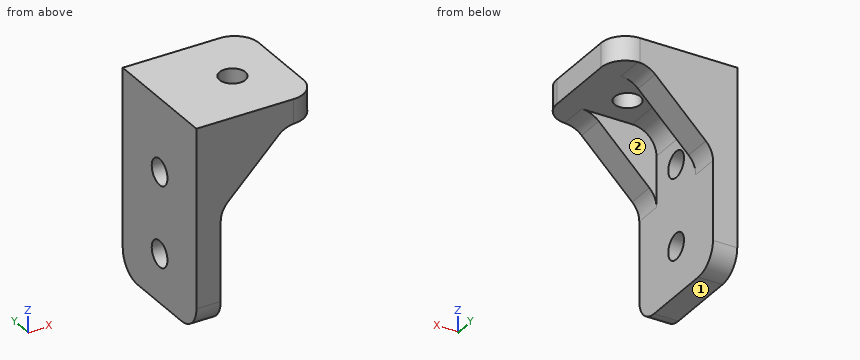
from build123d import *

# Parameters (mm, degrees)
SKETCH1_W           = 3
SKETCH1_H           = 22
SKETCH1_H_2         = 3
SKETCH1_W_2         = 12
BOSS_EXTRUDE1_DEPTH = 15
SKETCH2_R           = 1.6
CUT_EXTRUDE1_DEPTH  = 31.56141358
SKETCH3_R           = 1.6
CUT_EXTRUDE2_DEPTH  = 32.527765541
FILLET1_R           = 3
CHAMFER1_SIZE       = 8
SKETCH6_W           = 8
SKETCH6_H           = 8
CUT_EXTRUDE5_DEPTH  = 12
FILLET2_R           = 3
SKETCH7_W           = 15
SKETCH7_H           = 25
CUT_EXTRUDE6_DEPTH  = 33.787192713


with BuildPart() as part:
    # Sketch1 → Boss-Extrude1 (new body)
    with BuildSketch(Plane(origin=(0, 0, 0), x_dir=(1, 0, 0), z_dir=(0, 1, 0))):
        with Locations((1.5, 14)):
            Rectangle(SKETCH1_W, SKETCH1_H)
        with Locations((1.5, 1.5)):
            Rectangle(SKETCH1_W, SKETCH1_H_2)
        with Locations((9, 1.5)):
            Rectangle(SKETCH1_W_2, SKETCH1_H_2)
    extrude(amount=BOSS_EXTRUDE1_DEPTH)

    # Sketch2 → Cut-Extrude1 (cut, through all)
    with BuildSketch(Plane(origin=(0, 0, -3), x_dir=(-1, 0, 0), z_dir=(0, 0, -1))):
        with Locations((-9, 7.5)):
            Circle(SKETCH2_R)
    extrude(amount=-CUT_EXTRUDE1_DEPTH, mode=Mode.SUBTRACT)

    # Sketch3 → Cut-Extrude2 (cut, through all)
    with BuildSketch(Plane(origin=(3, 0, 0), x_dir=(0, 0, -1), z_dir=(1, 0, 0))):
        with Locations((9, 7.5)):
            Circle(SKETCH3_R)
        with Locations((19, 7.5)):
            Circle(SKETCH3_R)
    extrude(amount=-CUT_EXTRUDE2_DEPTH, mode=Mode.SUBTRACT)

    # Fillet1
    fillet1_edges = [part.edges().sort_by_distance(p)[0] for p in [
        (15, 15, -1.5),
        (1.5, 15, -25),
        (1.5, 0, -25),
        (15, 0, -1.5),
    ]]
    fillet(fillet1_edges, radius=FILLET1_R)

    # Chamfer1
    # the kernel refuses this chamfer: 8 mm, written as the material it adds along each edge
    with BuildSketch(Plane(origin=(3, 0, -3), x_dir=(-0.027495876610586382, 0, -0.9996219169112968), z_dir=(0, 1, 0))) as chamfer1_piece_1_section:
        Polygon((CHAMFER1_SIZE * 0.999621916911, -CHAMFER1_SIZE * 0.0274958766106), (-CHAMFER1_SIZE * 0.0274958766106, -CHAMFER1_SIZE * 0.999621916911), (0, 0), align=None)
    chamfer1_piece_1 = extrude(amount=15, mode=Mode.PRIVATE)
    chamfer1_piece_1 = chamfer1_piece_1 - Plane(origin=(5.584357769, 7.5, -9), x_dir=(0, 0, -1), z_dir=(1, 0, 0)) * Cylinder(1.6, 62, mode=Mode.PRIVATE)
    chamfer1_piece_1 = chamfer1_piece_1 - Plane(origin=(9, 7.5, -5.584358399), x_dir=(-1, 0, 0), z_dir=(0, 0, -1)) * Cylinder(1.6, 62, mode=Mode.PRIVATE)
    add(chamfer1_piece_1)

    # Sketch6 → Cut-Extrude5 (cut)
    with BuildSketch(Plane(origin=(15, 0, 0), x_dir=(0, 0, -1), z_dir=(1, 0, 0))):
        with Locations((7, 7.5)):
            Rectangle(SKETCH6_W, SKETCH6_H)
    extrude(amount=-CUT_EXTRUDE5_DEPTH, mode=Mode.SUBTRACT)

    # Fillet2
    fillet2_edges = [part.edges().sort_by_distance(p)[0] for p in [
        (3, 7.5, -3),
        (11, 1.75, -3),
        (3, 1.75, -11),
        (3, 13.25, -11),
        (11, 13.25, -3),
    ]]
    fillet(fillet2_edges, radius=FILLET2_R)

    # Mirror3: part across plane


with BuildPart() as part_1:
    add(part.part)
    add(part.part.mirror(Plane(origin=(0, 15, 0), x_dir=(0, 0, 1), z_dir=(-1, 0, 0))))

    # Sketch7 → Cut-Extrude6 (cut, through all)
    with BuildSketch(Plane.XZ):
        with Locations((-7.5, -12.5)):
            Rectangle(SKETCH7_W, SKETCH7_H)
    extrude(amount=-CUT_EXTRUDE6_DEPTH, mode=Mode.SUBTRACT)


solid = part_1.part
Can you work these out from the model? Positions are in its coordinate system, mm. Face numbers are marked on the shaded views. A direction names the side the tool comes from. Coordinates: 2 decimals unless noted, no trailing zeros. Write each loop counter-clockwise with the first axis right and the second up, starting at its lowest first coordinate (ties: lowest second). Pieces come first, ordered by that corner, then holes. Notation, with made-up numbers: (-31, -36) -> (-18, -36) arc R22 cw to (-18, -29) -> close; hole circle Ø9 at (3, 10.5). An arc over 180 degrees is marked (long way). Write each question's results on one line, items separated by ' | '. Start each with the question number.
Item 1: I'm going to push flat-ended pins straight in: P1, Ø6, axis at x = 7, y = 2, coming from the +Z side; P2, Ø4.5, axis at y = 9, z = -19, coming from the +X side; P3, Ø1.5, axis at x = 12.5, y = 7, coming from the -Z side; P4, Ø1.9, axis at y = 7.5, z = -19, coming from the +X side. Where does each tip first touch, or does it pass through?
Item 2: On a 3-axis mill with a long thin cutter (end or side, diameter ignored), from which of +Z, -Z, +X, -X, +Y, -Y can I reach the whole of each face in a straight line? I mean the marked faces 1 and 2. Say none if no direction works.
Item 3: If we section it at A-A, the plane z = -19: Write out the boundary of the cut face in (x, y).
Item 4: If we section it at D-D, the plane y = 9.5: Write out the boundary of the cut face in (x, z), and give its area (3 significant figures).
Item 5: If we section it at B-B, the plane x = 9: Write out the boundary of the cut face in (y, z), and give its area (3 significant figures).
Item 6: Please list where these lines run through material, in increasing order: probe 1 along Z at (x, y) = (1.6, 7.5); probe 2 along Y at (x, z) = (5.25, -3.75); probe 3 along Y at (x, z) = (2.35, -19).
Item 7: If we section it at C-C, the plane y = 7.5: Write out the boundary of the cut face in (x, z), and give its area (3 significant figures).
Answer block:
1) P1: z = 0 | P2: x = 3 | P3: z = -3 | P4: through
2) face 1: -Z, +X, -X, +Y, -Y | face 2: -Z, +X
3) outline: (0, 0) -> (3, 0) -> (3, 5.9) -> (0, 5.9) -> close; (0, 9.1) -> (3, 9.1) -> (3, 15) -> (0, 15) -> close
4) outline: (0, -25) -> (3, -25) -> (3, -6) arc R3 cw to (6, -3) -> (15, -3) -> (15, 0) -> (0, 0) -> close | area: 113 mm²
5) outline: (0, -5) -> (3.5, -5) -> (3.5, -3) -> (5.9, -3) -> (5.9, 0) -> (0, 0) -> close; (9.1, -3) -> (11.5, -3) -> (11.5, -5) -> (15, -5) -> (15, 0) -> (9.1, 0) -> close | area: 49.4 mm²
6) probe 1: -25 to -20.6, -17.4 to -10.6, -7.4 to 0 | probe 2: 0 to 3.5, 11.5 to 15 | probe 3: 0 to 5.9, 9.1 to 15
7) outline: (0, -25) -> (3, -25) -> (3, -20.6) -> (0, -20.6) -> close; (0, -17.4) -> (3, -17.4) -> (3, -10.6) -> (0, -10.6) -> close; (0, -7.4) -> (3, -7.4) -> (3, -6) arc R3 cw to (6, -3) -> (7.4, -3) -> (7.4, 0) -> (0, 0) -> close; (10.6, -3) -> (15, -3) -> (15, 0) -> (10.6, 0) -> close | area: 84.1 mm²
